The listing builds one solid part. Answer for the finished solid, in the listing's coordinates (mm). Face numbers are marked on the shaded views. A direction names the side the tool comes from. Give positions to 0.01 mm unless a question says otherwise; leave off trailing zeros. Write each loop counter-clockwise with the first axis right and the second up, starting at its lowest first coordinate (ties: lowest second). Pieces come first, ordered by that corner, then holes. Notation, with made-up numbers: (72, 89) -> (85, 89) arc R25 cw to (85, 108) -> close; hole circle Ø5 at (-7.75, 41.5). An arc over 180 degrees is marked (long way). Put each result on its own line as item: value. Start each with the question number.
1) For a pull along X with two mould halves and no side action, classify the marked faces 1, 2, 3 and 4 as released by +X, released by -X, zero draft, split by the parting line, or undercut.
2) Find the intervals of material crossed by line 1 along Y through (x, z) = (1.25, 1.9); line 2 along Y through (x, z) = (2.5, 1.8); line 3 along X through (y, z) = (-1, 1.8), in increasing order. Write a range as from..to.
3) For the marked faces 5 and 6, determine the directions among +Z, -Z, +X, -X, +Y, -Y from which every point of the face is accessible in a straight line to the end or side of a thin tool.
4) Flat-ended cylindrical pins translate along their axes: pin 1 Ø1 at (x, y) = (2, -2.5) entering from -Z; pin 2 Ø0.5 at (x, y) = (0, -3.5) entering from +Z. Find the tip coordinate at first contact, or state that the pin passes through.
5) A cutting plane is placed at B-B (y = 0). Write down the section's boundary in (x, z).
6) A cutting plane is placed at D-D (x = 1.25). Write down the section's boundary in (y, z).
7) A cutting plane is placed at C-C (z = 1.15). Give the number of separate pieces and of enclosed holes in the cut face, then the cut area to 3 significant figures.
8) A cutting plane is placed at A-A (x = 0). Write down the section's boundary in (y, z) (3 decimals).
from build123d import *

# Parameters (mm, degrees)
SZKIC1_R                    = 4.5
SZKIC1_R_2                  = 0.5
DODANIE_WYCI_GNI_CIE1_DEPTH = 2
SZKIC2_R                    = 0.5
WYTNIJ_WYCI_GNI_CIE2_DEPTH  = 1


with BuildPart() as part:
    # Szkic1 → Dodanie-wyciągnięcie1 (new body)
    with BuildSketch(Plane.XY):
        Circle(SZKIC1_R)
        Circle(SZKIC1_R_2, mode=Mode.SUBTRACT)
    extrude(amount=DODANIE_WYCI_GNI_CIE1_DEPTH)

    # Szkic2 → Wytnij-wyciągnięcie2 (cut)
    with BuildSketch(Plane.XY.offset(2)):
        with Locations((0, 3.625)):
            Circle(SZKIC2_R)
        with Locations((1.23982302, 3.40638575)):
            Circle(SZKIC2_R)
        with Locations((2.330105085, 2.776911106)):
            Circle(SZKIC2_R)
        with Locations((3.139342089, 1.8125)):
            Circle(SZKIC2_R)
        with Locations((3.569928105, 0.629474644)):
            Circle(SZKIC2_R)
        with Locations((3.569928105, -0.629474644)):
            Circle(SZKIC2_R)
        with Locations((3.139342089, -1.8125)):
            Circle(SZKIC2_R)
        with Locations((2.330105085, -2.776911106)):
            Circle(SZKIC2_R)
        with Locations((1.23982302, -3.40638575)):
            Circle(SZKIC2_R)
        with Locations((0, -3.625)):
            Circle(SZKIC2_R)
        with Locations((-1.23982302, -3.40638575)):
            Circle(SZKIC2_R)
        with Locations((-2.330105085, -2.776911106)):
            Circle(SZKIC2_R)
        with Locations((-3.139342089, -1.8125)):
            Circle(SZKIC2_R)
        with Locations((-3.569928105, -0.629474644)):
            Circle(SZKIC2_R)
        with Locations((-3.569928105, 0.629474644)):
            Circle(SZKIC2_R)
        with Locations((-3.139342089, 1.8125)):
            Circle(SZKIC2_R)
        with Locations((-2.330105085, 2.776911106)):
            Circle(SZKIC2_R)
        with Locations((-1.23982302, 3.40638575)):
            Circle(SZKIC2_R)
    extrude(amount=-WYTNIJ_WYCI_GNI_CIE2_DEPTH, mode=Mode.SUBTRACT)


solid = part.part
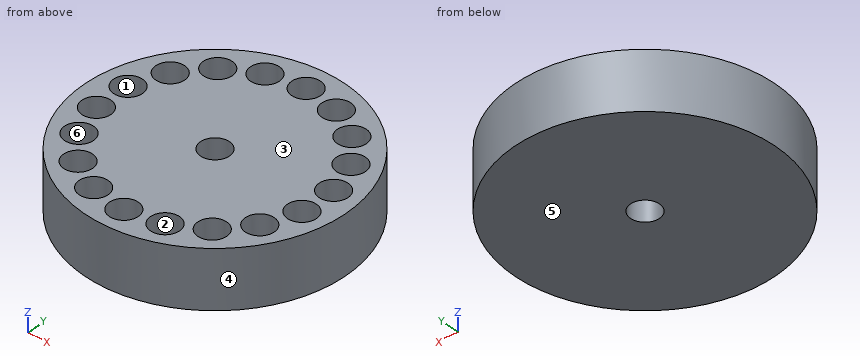
Reply:
1. face 1: undercut
1. face 2: undercut
1. face 3: zero draft
1. face 4: split by the parting line
2. line 1: y = -4.32..-3.91, -2.91..2.91, 3.91..4.32
2. line 2: y = -3.74..-3.25, -2.31..2.31, 3.25..3.74
2. line 3: x = -4.39..-3.91, -3.23..3.23, 3.91..4.39
3. face 5: -Z, +X, -X, +Y, -Y
3. face 6: +Z
4. pin 1: stops at z = 0
4. pin 2: stops at z = 1
5. outline: (-4.5, 0) -> (-0.5, 0) -> (-0.5, 2) -> (-4.5, 2) -> close; (0.5, 0) -> (4.5, 0) -> (4.5, 2) -> (0.5, 2) -> close
6. outline: (-4.32, 0) -> (4.32, 0) -> (4.32, 2) -> (3.91, 2) -> (3.91, 1) -> (2.91, 1) -> (2.91, 2) -> (-2.91, 2) -> (-2.91, 1) -> (-3.91, 1) -> (-3.91, 2) -> (-4.32, 2) -> close
7. separate pieces: 1
7. enclosed holes: 19
7. area: 48.7 mm2
8. outline: (-4.5, 0) -> (-0.5, 0) -> (-0.5, 2) -> (-3.125, 2) -> (-3.125, 1) -> (-4.125, 1) -> (-4.125, 2) -> (-4.5, 2) -> close; (0.5, 0) -> (4.5, 0) -> (4.5, 2) -> (4.125, 2) -> (4.125, 1) -> (3.125, 1) -> (3.125, 2) -> (0.5, 2) -> close
